Model file for the job. Use its own axes, mm. Give positions to 0.01 mm unless a question says otherwise; leave off trailing zeros. Loops run counter-clockwise (first coordinate to the right, second up) from the corner with the lowest first, then second, coordinate; pieces in that order, holes last. Notation, with made-up numbers: M 66.5,-10 L 125.5,-10 A30 cw 125.5,20 Z; hole C -40,66.25 d9. An arc over 180 degrees is marked long. Use CSV: the item, a comma, the result in double quotes. Start each with the question number.
(1) Slice it at B-B on x = 24. List the corners of the cut face in (y, z), and give its area (4 significant figures).
(2) Wall check: line 1 along Z through (x, y) = (-25, -12); line 2 along Y through (x, z) = (29.5, 127); line 3 along Y through (x, z) = (-17, 814). Give the ranges that are in metal, low to high. Write a range as from..to.
(3) Flat gauge pins, fed straight in: P1, Ø16, axis at x = 18, y = 22.5, coming from the +Z side; P2, Ø10, axis at x = -18, z = 846, coming from the -Y side; P3, Ø6, axis at y = 21.5, z = 837, coming from the +X side; P4, Ø16, axis at x = -18.5, y = -23.5, coming from the +Z side. Where does each tip first touch, or does it go through?
(4) Slice it at C-C on y = 17.5. List the corners of the cut face in (x, z), and give its area (3 significant figures).
(5) Slice it at A-A on y = -22. List the corners of the cut face in (x, z).
```python
from build123d import *

# Parameters (mm, degrees)
F1_W      = 100
F1_H      = 100
F3_DEPTH  = 900
F4_W      = 20
F4_H      = 75
F5_DEPTH  = 50
F6_W      = 20
F6_H      = 75
F7_DEPTH  = 50
F9_DEPTH  = 100
F12_W     = 50
F12_H     = 20
F12_W_2   = 20
F12_H_2   = 50
F13_DEPTH = 87.5
F15_DEPTH = 100


with BuildPart() as f3:
    # F1 (on Top) → F3 (new body)
    with BuildSketch(Plane.XY):
        Rectangle(F1_W, F1_H)
    extrude(amount=F3_DEPTH)

    # F4 (on face) → F5 (cut)
    with BuildSketch(Plane.YZ.offset(50)):
        with Locations((17.5, 150)):
            Rectangle(F4_W, F4_H)
    extrude(amount=-F5_DEPTH, mode=Mode.SUBTRACT)

    # F6 (on face) → F7 (cut)
    with BuildSketch(Plane.XZ.offset(50)):
        with Locations((-17.5, 150)):
            Rectangle(F6_W, F6_H)
    extrude(amount=-F7_DEPTH, mode=Mode.SUBTRACT)


with BuildPart() as f9:
    # F8 (on Top) → F9 (new body)
    with BuildSketch(Plane.XY):
        Polygon((50, -40), (40, -50), (50, -50), align=None)
    extrude(amount=F9_DEPTH)


with BuildPart() as f9_1:
    # F10: moved
    add(f9.part.moved(Location((0, 0, 100))))


with BuildPart() as f3_1:
    add(f3.part)

    # F11: cut F9
    add(f9_1.part, mode=Mode.SUBTRACT)

    # F12 (on face) → F13 (cut)
    with BuildSketch(Plane.XY.offset(900)):
        with Locations((25, 17.5)):
            Rectangle(F12_W, F12_H)
        with Locations((-17.5, -25)):
            Rectangle(F12_W_2, F12_H_2)
    extrude(amount=-F13_DEPTH, mode=Mode.SUBTRACT)

    # F12 (on face) → F15 (cut)
    with BuildSketch(Plane.XY.offset(900)):
        Polygon((50, -50), (50, -40), (40, -50), align=None)
    extrude(amount=-F15_DEPTH, mode=Mode.SUBTRACT)


solid = f3_1.part
```
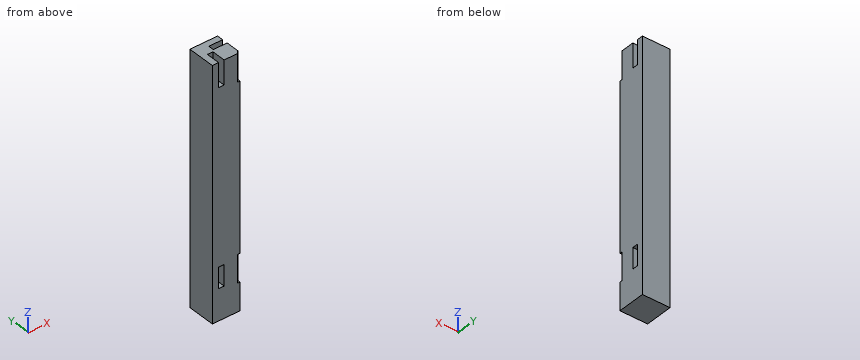
Reply:
1,outline,"M -50,0 L 50,0 L 50,900 L 27.5,900 L 27.5,812.5 L 7.5,812.5 L 7.5,900 L -50,900 Z; hole M 7.5,112.5 L 27.5,112.5 L 27.5,187.5 L 7.5,187.5 Z"
1,area,"86,750 mm^2"
2,line 1,"z = 0..112.5, 187.5..812.5"
2,line 2,"y = -50..7.5, 27.5..50"
2,line 3,"y = 0..50"
3,P1,"stops at z = 900"
3,P2,"stops at y = 0"
3,P3,"stops at x = 0"
3,P4,"stops at z = 812.5"
4,outline,"M -50,0 L 50,0 L 50,112.5 L 0,112.5 L 0,187.5 L 50,187.5 L 50,812.5 L 0,812.5 L 0,900 L -50,900 Z"
4,area,"81,900 mm^2"
5,outline,"M -50,0 L 50,0 L 50,900 L -7.5,900 L -7.5,812.5 L -27.5,812.5 L -27.5,900 L -50,900 Z; hole M -27.5,112.5 L -7.5,112.5 L -7.5,187.5 L -27.5,187.5 Z"
